Here's the drawing with two shaded views (mm, measured from the low corner). I have some questions. Round coordinates to 2 decimals unless told otherwise and drop trailing zeros. Loops run counter-clockwise (first coordinate to the right, second up) from the corner with the lowest first, then second, coordinate; pieces in that order, holes last. Notation, with made-up numbers: (54, -22.5) - (63, -22.5) arc R22 cw to (63, -16.5) - close; hole circle Ø6 at (-33.5, 64.25). An arc over 180 degrees is marked (long way). Answer as CSV lines item,"result".
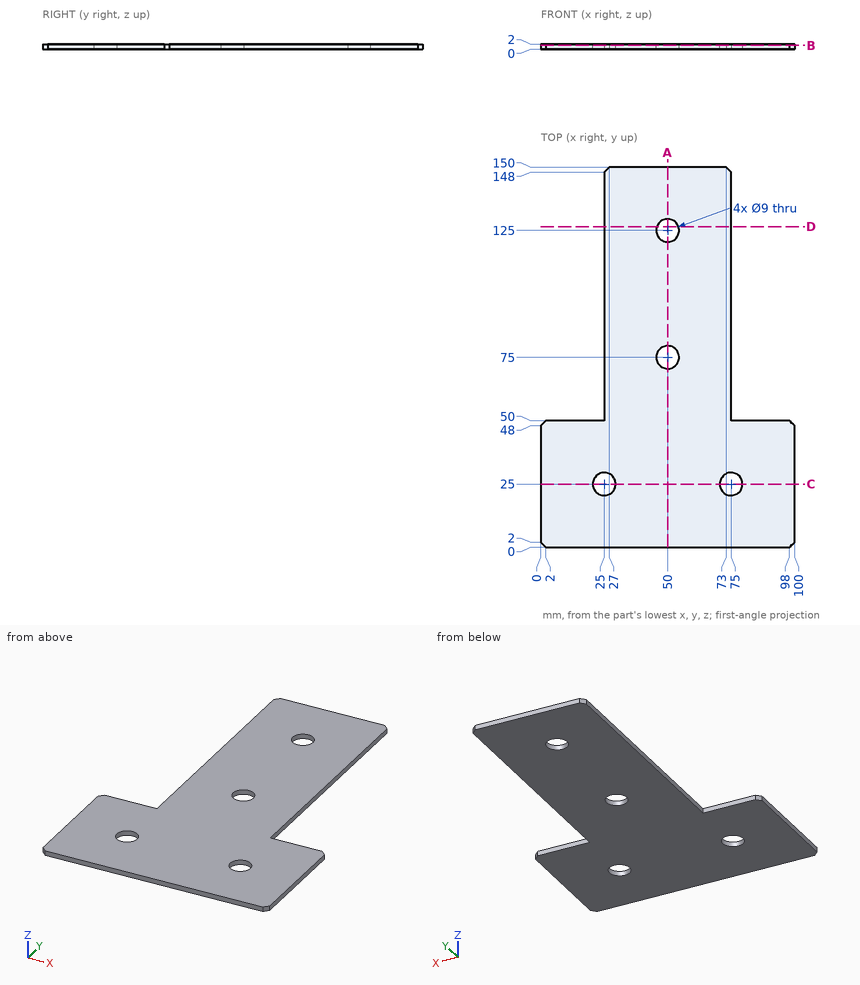
Q1. Imagine slicing it at C-C (y = 25). Write out the boundary of the cut face in (x, z).
Checks:
outline,"(0, 0) - (20.5, 0) - (20.5, 2) - (0, 2) - close; (29.5, 0) - (70.5, 0) - (70.5, 2) - (29.5, 2) - close; (79.5, 0) - (100, 0) - (100, 2) - (79.5, 2) - close"
Q2. I'm going to push flat-ended pins straight in: pin 1 Ø1 at (y, z) = (111.5, 0.5) entering from -X; pin 2 Ø14.5 at (x, y) = (25, 25) entering from -Z; pin 3 Ø7 at (x, y) = (50, 75) entering from +Z; pin 4 Ø1 at (x, z) = (88, 1) entering from +Y. Where does each tip first touch, or does it pass through?
Checks:
pin 1,"x = 25"
pin 2,"z = 0"
pin 3,"through"
pin 4,"y = 50"
Q3. Imagine slicing it at A-A (x = 50). Write out the boundary of the cut face in (y, z).
Checks:
outline,"(0, 0) - (70.5, 0) - (70.5, 2) - (0, 2) - close; (79.5, 0) - (120.5, 0) - (120.5, 2) - (79.5, 2) - close; (129.5, 0) - (150, 0) - (150, 2) - (129.5, 2) - close"
Q4. Imagine slicing it at B-B (z = 1.45). Write out the boundary of the cut face in (x, y), then the cut area to 3 significant figures.
Checks:
outline,"(0, 2) - (2, 0) - (98, 0) - (100, 2) - (100, 48) - (98, 50) - (75, 50) - (75, 148) - (73, 150) - (27, 150) - (25, 148) - (25, 50) - (2, 50) - (0, 48) - close; hole circle Ø9 at (25, 25); hole circle Ø9 at (50, 75); hole circle Ø9 at (50, 125); hole circle Ø9 at (75, 25)"
area,"9,730 mm²"
Q5. Imagine slicing it at D-D (y = 126.5). Write out the boundary of the cut face in (x, z), then the cut area to 3 significant figures.
Checks:
outline,"(25, 0) - (45.76, 0) - (45.76, 2) - (25, 2) - close; (54.24, 0) - (75, 0) - (75, 2) - (54.24, 2) - close"
area,"83.0 mm²"
Q6. If I drill on line 1 along Y through (x, z) = (50, 1.3); line 2 along X through (y, z) = (125, 0.8); line 3 along X through (y, z) = (23.5, 1.7), over which ranges is the centre line in solid material (lowest first)? Write a range as [from, to].
Checks:
line 1,"[0, 70.5], [79.5, 120.5], [129.5, 150]"
line 2,"[25, 45.5], [54.5, 75]"
line 3,"[0, 20.76], [29.24, 70.76], [79.24, 100]"
